Autodesk Inventor part; units mm, degrees
ref_plane "YZ Plane" through (0, 0, 0) normal (1, 0, 0) x (0, 1, 0)
ref_plane "XZ Plane" through (0, 0, 0) normal (0, 1, 0) x (-1, 0, 0)
ref_plane "XY Plane" through (0, 0, 0) normal (0, 0, 1) x (1, 0, 0)
sketch "Szkic1" plane through (0, 0, 0) normal (0, 1, 0) x (-1, 0, 0)
  circle A0 centre (0, 0) radius 5
  dimension "d0" = 10
extrude "Wyciągnięcie proste1" add sketch "Szkic1" along normal blind 20
sketch "Szkic2" plane through (0, 0, 0) normal (0, -1, 0) x (1, 0, 0)
  circle A0 centre (0, 0) radius 10
  dimension "d3" = 20
extrude "Wyciągnięcie proste2" add sketch "Szkic2" against normal blind 5
sketch "Szkic3" plane through (0, 20, 0) normal (0, 1, 0) x (1, 0, 0)
  circle A0 centre (0, 0) radius 10
extrude "Wyciągnięcie proste3" add sketch "Szkic3" along normal blind 5
properties part number "dopodniesienia1"
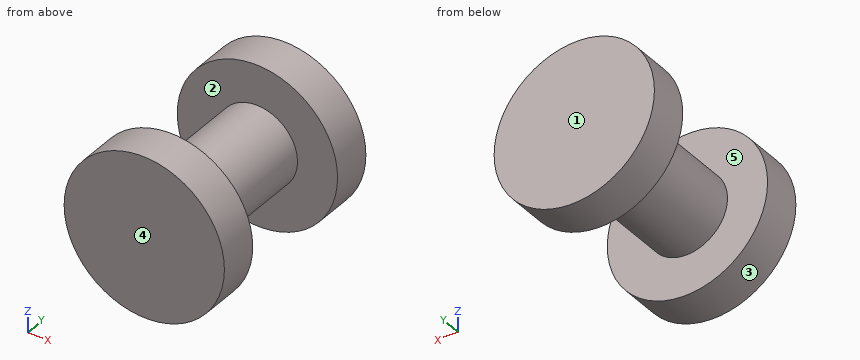
Geometry check sheet. Reference: the model listing, model coordinates, mm. Face numbers are marked on the shaded views. A direction names the side the tool comes from. Give positions to 0.01 mm unless a question says otherwise; leave off trailing zeros. Write each loop counter-clockwise with the first axis right and the second up, starting at its lowest first coordinate (ties: lowest second). Pieces come first, ordered by that corner, then holes. Notation, with made-up numbers: (46, 50) - (54, 50) arc R18 ccw to (54, 62) - close; hole circle Ø9 at (24.5, 57). An arc over 180 degrees is marked (long way). Use a Markdown table: item, result.
Q1. Section check D-D, the plane x = 0. Enter the section's corners in (y, z).
Computed:
| item | result |
|---|---|
| outline | (0, -10) - (5, -10) - (5, -5) - (20, -5) - (20, -10) - (25, -10) - (25, 10) - (20, 10) - (20, 5) - (5, 5) - (5, 10) - (0, 10) - close |
Q2. Section check B-B, the plane x = 5.75. Enter the section's corners in (y, z).
Computed:
| item | result |
|---|---|
| outline | (0, -8.18) - (5, -8.18) - (5, 8.18) - (0, 8.18) - close; (20, -8.18) - (25, -8.18) - (25, 8.18) - (20, 8.18) - close |
Q3. Thickness scan on L1, parallel to Y at x = 5, z = 5.75; L2, parallel to Z at x = 8.25, y = 2; L3, parallel to Z at x = -3, y = 19. Record the ranges inside material, lowest first. Write a range as [from, to].
Computed:
| item | result |
|---|---|
| L1 | y = [0, 5], [20, 25] |
| L2 | z = [-5.65, 5.65] |
| L3 | z = [-4, 4] |
Q4. Section check C-C, the plane z = 0. Enter the section's corners in (x, y), then the cut area to 3 significant figures.
Computed:
| item | result |
|---|---|
| outline | (-10, 0) - (10, 0) - (10, 5) - (5, 5) - (5, 20) - (10, 20) - (10, 25) - (-10, 25) - (-10, 20) - (-5, 20) - (-5, 5) - (-10, 5) - close |
| area | 350 mm² |
Q5. Section check A-A, the plane z = 8.25. Enter the section's corners in (x, y), then the cut area to 3 significant figures.
Computed:
| item | result |
|---|---|
| outline | (-5.65, 0) - (5.65, 0) - (5.65, 5) - (-5.65, 5) - close; (-5.65, 20) - (5.65, 20) - (5.65, 25) - (-5.65, 25) - close |
| area | 113 mm² |
Q6. Draft check along Y on the marked faces 1, 2 and 3. Enter one of: pulls with the +Y half, pulls with the -Y half, needs draft (parallel to the pull), parting line crosses it, or undercut.
Computed:
| item | result |
|---|---|
| face 1 | pulls with the +Y half |
| face 2 | undercut |
| face 3 | needs draft |
Q7. Go/stop test with flat-tipped pins: P1, Ø2, axis at x = 4, y = 3, coming from the -Z side; P2, Ø12, axis at y = 15.5, z = 6, coming from the +X side; P3, Ø6, axis at x = -5, y = 19, coming from the +Z side. Record where each tip stops, or that it passes through.
Computed:
| item | result |
|---|---|
| P1 | stops at z = -9.54 |
| P2 | stops at x = 9.79 |
| P3 | stops at z = 9.76 |
Q8. Set-up check for the marked faces 4 and 5: record each of +Z, -Z, +X, -X, +Y, -Y from which the full face is reachable in a straight line by a thin tool's end or side.
Computed:
| item | result |
|---|---|
| face 4 | +Z, -Z, +X, -X, -Y |
| face 5 | none |
